Part print with two shaded views. Sizes in mm from the minimum x, y, z corner. A direction names the side the tool comes from. Round coordinates to 2 decimals unless told otherwise and drop trailing zeros. Write each loop counter-clockwise with the first axis right and the second up, starting at its lowest first coordinate (ties: lowest second). Pieces come first, ordered by that corner, then holes. Notation, with made-up numbers: (2.25, 66) -> (45.25, 66) arc R35 cw to (45.25, 103) -> close; hole circle Ø1 at (50, 67). An arc over 180 degrees is marked (long way). Return JSON: item names as keys, results as strings. Group by question number.
(1) Drop flat-ended pins along their axis: pin 1 Ø5 at (y, z) = (21.5, 12.5) entering from -X (3 decimals); pin 2 Ø9.5 at (x, z) = (23.5, 15.5) entering from +Y; pin 3 Ø1 at (x, z) = (25.5, 17.5) entering from +Y; pin 4 Ø4.5 at (x, y) = (26, 14.5) entering from -Z. Give the stop position or say it passes through.
(2) Drill centre lines: L1, parallel to Y at x = 32.5, z = 14.5; L2, parallel to X at y = 14.5, z = 12.5 (3 decimals); L3, parallel to Z at x = 30, y = 17.5. Where is each one in solid material? Low to high. Write a range as from..to.
(3) Saw through at B-B (z = 14.48). List the corners of the cut face in (x, y) (3 decimals).
(4) Saw through at A-A (x = 25). List the corners of the cut face in (y, z), plus the area to 3 significant figures.
(5) Saw through at D-D (x = 34.5). List the corners of the cut face in (y, z).
(6) Saw through at C-C (y = 15). List the corners of the cut face in (x, z) (3 decimals).
(7) Tool access for the marked faces 1, 2 and 3: list every direction of +Z, -Z, +X, -X, +Y, -Y with a clear straight run to the whole face (end or side of a thin tool).
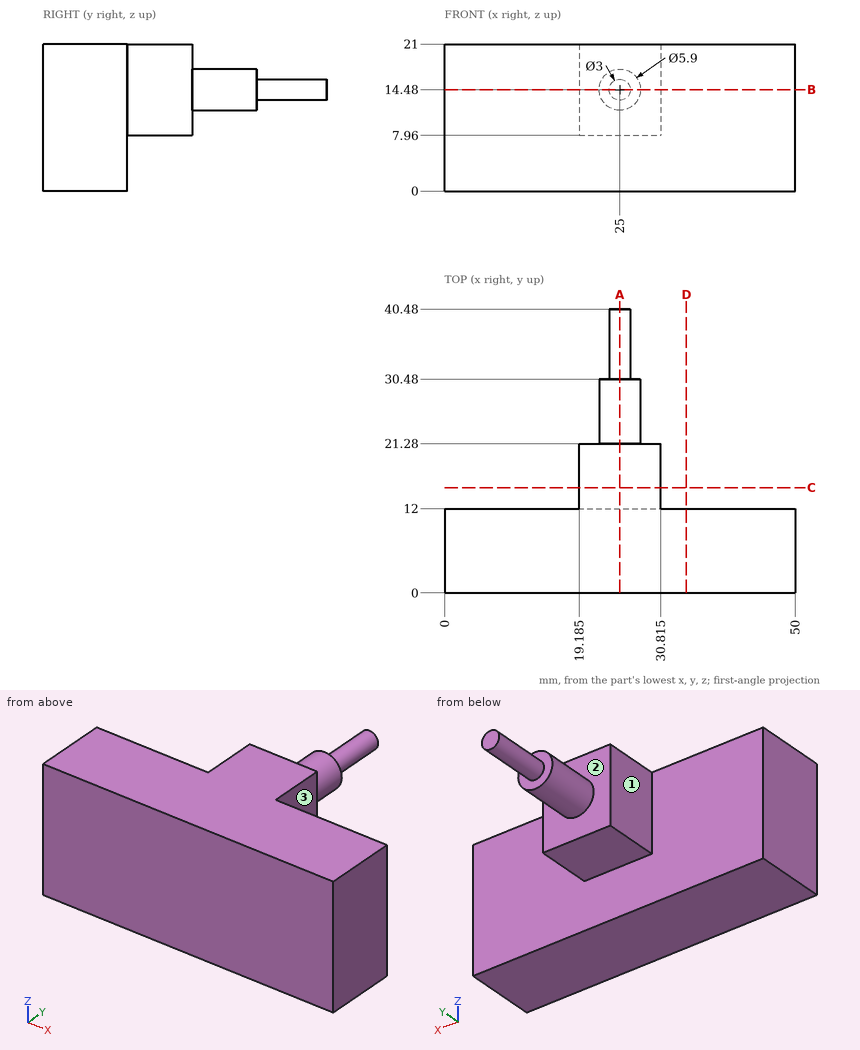
Computed values:
{
 "1": {"pin 1": "x = 19.185", "pin 2": "y = 40.48", "pin 3": "y = 30.48", "pin 4": "z = 7.96"},
 "2": {"L1": "0..12", "L2": "19.185..30.815", "L3": "7.96..21"},
 "3": {"outline": "(0, 0) -> (50, 0) -> (50, 12) -> (30.815, 12) -> (30.815, 21.28) -> (27.95, 21.28) -> (27.95, 30.48) -> (26.5, 30.48) -> (26.5, 40.48) -> (23.5, 40.48) -> (23.5, 30.48) -> (22.05, 30.48) -> (22.05, 21.28) -> (19.185, 21.28) -> (19.185, 12) -> (0, 12) -> close"},
 "4": {"outline": "(0, 0) -> (12, 0) -> (12, 7.96) -> (21.28, 7.96) -> (21.28, 11.53) -> (30.48, 11.53) -> (30.48, 12.98) -> (40.48, 12.98) -> (40.48, 15.98) -> (30.48, 15.98) -> (30.48, 17.43) -> (21.28, 17.43) -> (21.28, 21) -> (0, 21) -> close", "area": "457 mm2"},
 "5": {"outline": "(0, 0) -> (12, 0) -> (12, 21) -> (0, 21) -> close"},
 "6": {"outline": "(19.185, 7.96) -> (30.815, 7.96) -> (30.815, 21) -> (19.185, 21) -> close"},
 "7": {"face 1": "+Z, -Z, -X, +Y", "face 2": "+Y", "face 3": "+Z, -Z, +X, +Y"}
}
